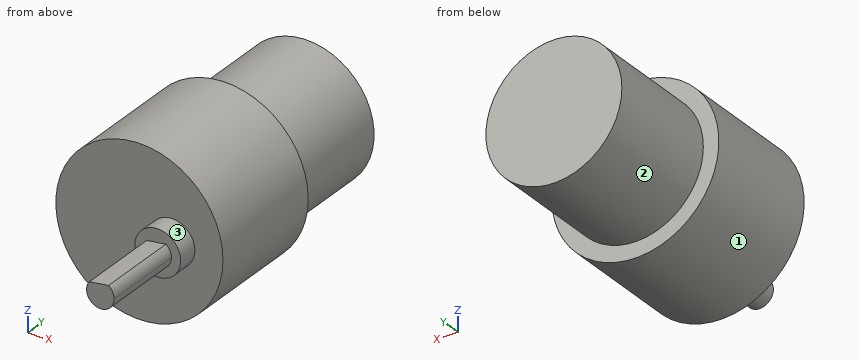
from build123d import *

# Parameters (mm, degrees)
F0_R     = 18.25
F1_DEPTH = 26.9
F4_DEPTH = 4.5
F6_DEPTH = 18.1
F7_R     = 14.854724
F8_DEPTH = 25.7


with BuildPart() as f1:
    # F0 (on Front) → F1 (new body)
    with BuildSketch(Plane.XZ):
        Circle(F0_R)
    extrude(amount=F1_DEPTH)

    # F3 (on face) → F4 (join)
    with BuildSketch(Plane.XZ.offset(26.9)):
        with BuildLine():
            ThreePointArc((10.116222, 0), (7.116222, 3), (4.116222, 0))
            Line((4.116222, 0), (10.116222, 0))
        make_face()
        with BuildLine():
            Line((10.116222, 0), (4.116222, 0))
            ThreePointArc((4.116222, 0), (7.116222, -3), (10.116222, 0))
        make_face()
        with BuildLine():
            Line((4.116222, 0), (2.116222, 0))
            ThreePointArc((2.116222, 0), (7.116222, -5), (12.116222, 0))
            Line((12.116222, 0), (10.116222, 0))
            ThreePointArc((10.116222, 0), (7.116222, -3), (4.116222, 0))
        make_face()
        with BuildLine():
            ThreePointArc((12.116222, 0), (7.116222, 5), (2.116222, 0))
            Line((2.116222, 0), (4.116222, 0))
            ThreePointArc((4.116222, 0), (7.116222, 3), (10.116222, 0))
            Line((10.116222, 0), (12.116222, 0))
        make_face()
    extrude(amount=F4_DEPTH)

    # F5 (on face) → F6 (join)
    with BuildSketch(Plane.XZ.offset(31.4)):
        Polygon((7.116222, 0), (8.912379, 2.402878), (4.713345, 1.796157), align=None)
        with BuildLine():
            ThreePointArc((4.713345, 1.796157), (6.169817, -2.846808), (10.116222, 0))
            ThreePointArc((10.116222, 0), (9.798429, 1.343788), (8.912379, 2.402878))
            Line((8.912379, 2.402878), (7.116222, 0))
            Line((7.116222, 0), (4.713345, 1.796157))
        make_face()
    extrude(amount=F6_DEPTH)

    # F7 (on face) → F8 (join)
    with BuildSketch(Plane(origin=(0, 0, 0), x_dir=(-1, 0, 0), z_dir=(0, 1, 0))):
        Circle(F7_R)
    extrude(amount=F8_DEPTH)


solid = f1.part
CAD build for the part. Positions are in the model's coordinates, mm. Face numbers are marked on the shaded views. A direction names the side the tool comes from. Coordinates: 2 decimals unless noted, no trailing zeros. Write each loop counter-clockwise with the first axis right and the second up, starting at its lowest first coordinate (ties: lowest second). Pieces come first, ordered by that corner, then holes. Notation, with made-up numbers: (76.5, -34.75) - (129.5, -34.75) arc R19 ccw to (129.5, -9.75) - close; hole circle Ø9 at (27.5, 35). An arc over 180 degrees is marked (long way). Use a Markdown table: item, result. Add a question column.
Item 1: Drill centre lines: L1, parallel to Y at x = 6.5, z = 7; L2, parallel to Y at x = 9.5, z = -2; L3, parallel to Z at x = -6.5, y = 21.5. Where is each one in solid material? Low to high. Write a range as from..to.
Item 2: 3-axis set-ups, long thin cutter, end or side, ignore diameter. For the marked faces 1, 2 and 3: which of +Z, -Z, +X, -X, +Y, -Y reach the whole face in a straight line?
Item 3: Flat gauge pins, fed straight in: pin 1 (2 mm diameter, centred on y = -38.5, z = 1.5, fed in from -X); pin 2 (12 mm diameter, centred on x = 14.5, y = 7, fed in from -Z); pin 3 (2 mm diameter, centred on x = -6, z = 0, fed in from -Y). Where does each tip first touch, or does it go through?
Item 4: Band-saw the part on B-B, the plane z = -10. Give the cut face in (x, y).
Item 5: Band-saw the part on C-C, the plane y = -34.5. Give the cut face in (x, z), and give its area (3 significant figures).
Item 6: Band-saw the part on A-A, the plane x = 0. Give the cut face in (y, z).
Item 7: Band-saw the part on D-D, the plane y = 11.5. Give the cut face in (x, z).
Numbers:
| question | item | result |
|---|---|---|
| 1 | L1 | -26.9..25.7 |
| 1 | L2 | -31.4..25.7 |
| 1 | L3 | -13.36..13.36 |
| 2 | face 1 | +Y, -Y |
| 2 | face 2 | +Y |
| 2 | face 3 | -Y |
| 3 | pin 1 | x = 4.16 |
| 3 | pin 2 | z = -12.18 |
| 3 | pin 3 | y = -26.9 |
| 4 | outline | (-15.27, -26.9) - (15.27, -26.9) - (15.27, 0) - (10.98, 0) - (10.98, 25.7) - (-10.98, 25.7) - (-10.98, 0) - (-15.27, 0) - close |
| 5 | outline | (4.71, 1.8) arc R3 ccw (long way) to (10.12, 0) arc R3 ccw to (8.91, 2.4) - close |
| 5 | area | 25.7 mm2 |
| 6 | outline | (-26.9, -18.25) - (0, -18.25) - (0, -14.85) - (25.7, -14.85) - (25.7, 14.85) - (0, 14.85) - (0, 18.25) - (-26.9, 18.25) - close |
| 7 | outline | circle Ø29.71 at (0, 0) |
